The figure shows three views and two pictorial views of one solid part (mm, origin at its lowest corner). Answer the questions. Coordinates: 2 decimals unless noted, no trailing zeros. Write each loop counter-clockwise with the first axis right and the second up, starting at its lowest first coordinate (ties: lowest second). Pieces come first, ordered by that corner, then holes. Notation, with made-up numbers: M -3,47 L 54,47 A22 cw 54,67 Z; hole C 25.25,61 d3. An arc over 180 degrees is marked long. Write item = value, one per line.
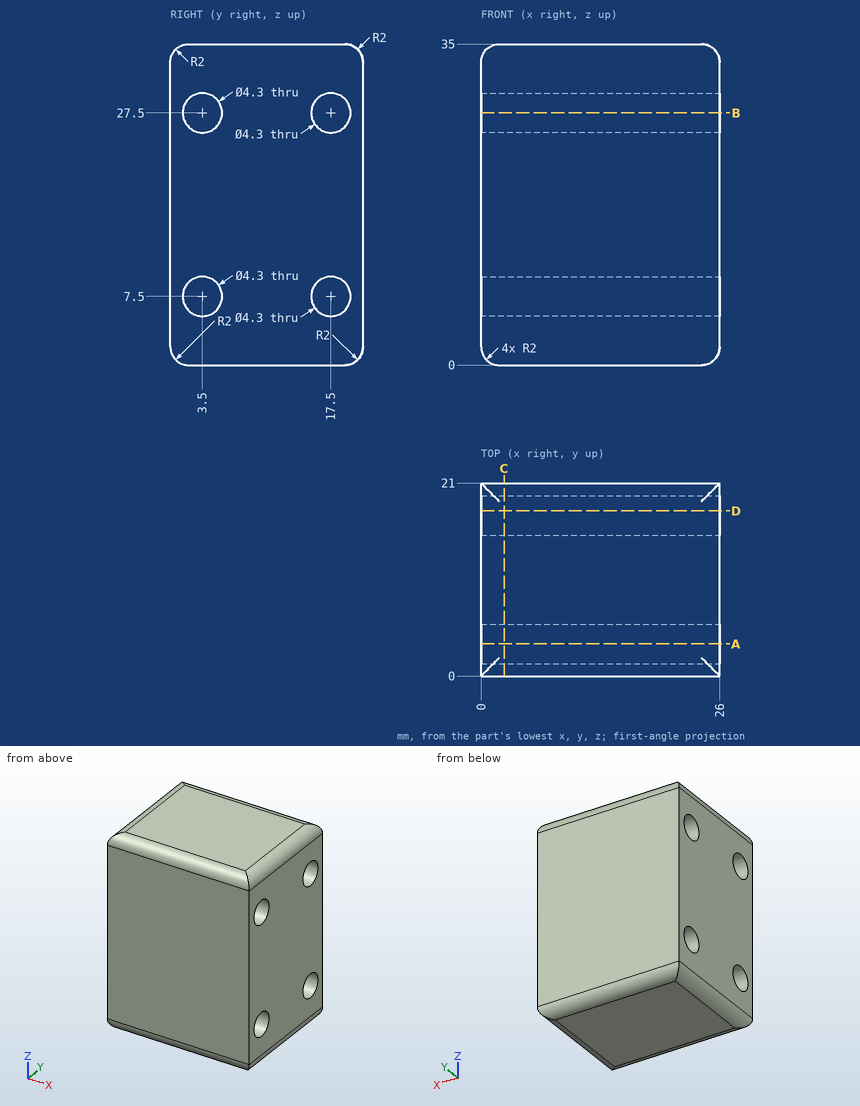
Item 1: Find section B-B (z = 27.5). Determine the outline of the cut face in (x, y).
Worked answers:
outline = M 0,0 L 26,0 L 26,1.35 L 0,1.35 Z; M 0,5.65 L 26,5.65 L 26,15.35 L 0,15.35 Z; M 0,19.65 L 26,19.65 L 26,21 L 0,21 Z
Item 2: Consider line 1 along Y through (x, z) = (9.5, 27.5); line 2 along Z through (x, y) = (14.25, 16.25); line 3 along Z through (x, y) = (12.25, 5). Determine where each line is inside the solid, lowest interval first. Write a range as from..to.
Worked answers:
line_1 = 0..1.35, 5.65..15.35, 19.65..21
line_2 = 0..5.75, 9.25..25.75, 29.25..35
line_3 = 0..5.96, 9.04..25.96, 29.04..35
Item 3: Flat-ended cylindrical pins translate along their axes: pin 1 (5.5 mm diameter, centred on y = 3.5, z = 27.5, fed in from -X); pin 2 (2.5 mm diameter, centred on y = 17.5, z = 27.5, fed in from -X) (1 decimal). Find the tip coordinate at first contact, or state that the pin passes through.
Worked answers:
pin_1 = 0
pin_2 = through
Item 4: Find section A-A (y = 3.5). Determine the outline of the cut face in (x, z), and give its area (3 significant figures).
Worked answers:
outline = M 0,2 A2 ccw 2,0 L 24,0 A2 ccw 26,2 L 26,5.35 L 0,5.35 Z; M 0,9.65 L 26,9.65 L 26,25.35 L 0,25.35 Z; M 0,29.65 L 26,29.65 L 26,33 A2 ccw 24,35 L 2,35 A2 ccw 0,33 Z
area = 683 mm²
Item 5: Find section C-C (x = 2.5). Determine the outline of the cut face in (y, z), and give its area (3 significant figures).
Worked answers:
outline = M 0,2 A2 ccw 2,0 L 19,0 A2 ccw 21,2 L 21,33 A2 ccw 19,35 L 2,35 A2 ccw 0,33 Z; hole C 3.5,7.5 d4.3; hole C 3.5,27.5 d4.3; hole C 17.5,7.5 d4.3; hole C 17.5,27.5 d4.3
area = 673 mm²
Item 6: Find section D-D (y = 18). Determine the outline of the cut face in (x, z), and give its area (3 significant figures).
Worked answers:
outline = M 0,2 A2 ccw 2,0 L 24,0 A2 ccw 26,2 L 26,5.41 L 0,5.41 Z; M 0,9.59 L 26,9.59 L 26,25.41 L 0,25.41 Z; M 0,29.59 L 26,29.59 L 26,33 A2 ccw 24,35 L 2,35 A2 ccw 0,33 Z
area = 689 mm²
